Model file for the job. Use its own axes, mm. Coordinates: 2 decimals unless noted, no trailing zeros. Loops run counter-clockwise (first coordinate to the right, second up) from the corner with the lowest first, then second, coordinate; pieces in that order, holes last.
Autodesk Inventor part; units mm, degrees
ref_plane "YZ Plane" through (0, 0, 0) normal (1, 0, 0) x (0, 1, 0)
ref_plane "XZ Plane" through (0, 0, 0) normal (0, 1, 0) x (-1, 0, 0)
ref_plane "XY Plane" through (0, 0, 0) normal (0, 0, 1) x (1, 0, 0)
sketch "Parede_lateral_1" plane through (0, 0, 0) normal (0, 1, 0) x (-1, 0, 0)
  line L0 (0, 0) -> (-95, 0)
  line L1 (-95, 0) -> (-95, -52)
  line L2 (-95, -52) -> (0, -52)
  line L3 (0, -52) -> (0, 0)
  dimension "d0" = 95
  dimension "d1" = 52
extrude "Extrusão1" add sketch "Parede_lateral_1" along normal blind 3
sketch "Esboço4" plane through (0, 3, 0) normal (0, 1, 0) x (1, 0, 0)
  line L0 (0, 52) -> (0, 0)
  line L1 (0, 42) -> (3, 42)
  line L2 (3, 42) -> (3, 32)
  line L3 (3, 32) -> (0, 32)
  line L4 (0, 32) -> (0, 42)
  line L5 (0, 20) -> (3, 20)
  line L6 (3, 20) -> (3, 10)
  line L7 (3, 10) -> (0, 10)
  line L8 (0, 10) -> (0, 20)
  line L9 (95, 0) -> (95, 52)
  line L10 (0, 0) -> (95, 0)
  line L11 (95, 42) -> (92, 42)
  line L12 (92, 42) -> (92, 32)
  line L13 (92, 32) -> (95, 32)
  line L14 (95, 32) -> (95, 42)
  line L15 (95, 20) -> (92, 20)
  line L16 (92, 20) -> (92, 10)
  line L17 (92, 10) -> (95, 10)
  line L18 (95, 10) -> (95, 20)
  line L19 (10, 0) -> (20, 0)
  line L20 (20, 0) -> (20, -3)
  line L21 (20, -3) -> (10, -3)
  line L22 (10, -3) -> (10, 0)
  line L23 (42.5, 0) -> (52.5, 0)
  line L24 (52.5, 0) -> (52.5, -3)
  line L25 (52.5, -3) -> (42.5, -3)
  line L26 (42.5, -3) -> (42.5, 0)
  line L27 (75, 0) -> (85, 0)
  line L28 (85, 0) -> (85, -3)
  line L29 (85, -3) -> (75, -3)
  line L30 (75, -3) -> (75, 0)
  point P0 (1.5, 42)
  point P1 (1.5, 10)
  dimension "d37" = 3
  dimension "d38" = 10
  dimension "d39" = 3
  dimension "d40" = 10
  dimension "d46" = 10
  dimension "d47" = 3
  dimension "d49" = 3
extrude "Extrusão4" add sketch "Esboço4" against normal blind 3 contours L10 L28 L29 L30 | L10 L24 L25 L26 | L10 L20 L21 L22
sketch "Esboço5" plane through (0, 3, 0) normal (0, 1, 0) x (1, 0, 0)
  line L0 (0, 52) -> (0, 0)
  line L1 (0, 10) -> (3, 10)
  line L2 (3, 10) -> (3, 20)
  line L3 (3, 20) -> (0, 20)
  line L4 (0, 20) -> (0, 10)
  line L5 (0, 32) -> (3, 32)
  line L6 (3, 32) -> (3, 42)
  line L7 (3, 42) -> (0, 42)
  line L8 (0, 42) -> (0, 32)
  line L9 (95, 52) -> (0, 52)
  line L10 (0, 0) -> (10, 0)
  line L11 (95, 0) -> (95, 52)
  line L12 (95, 42) -> (92, 42)
  line L13 (92, 42) -> (92, 32)
  line L14 (92, 32) -> (95, 32)
  line L15 (95, 32) -> (95, 42)
  line L16 (95, 20) -> (92, 20)
  line L17 (92, 20) -> (92, 10)
  line L18 (92, 10) -> (95, 10)
  line L19 (95, 10) -> (95, 20)
  point P0 (10, 52)
  point P1 (1.5, 42)
  point P2 (1.5, 10)
  dimension "d52" = 3
  dimension "d53" = 10
  dimension "d54" = 3
  dimension "d55" = 10
  dimension "d56" = 10
  dimension "d57" = 10
  dimension "d58" = 3
extrude "Extrusão5" cut sketch "Esboço5" against normal blind 3
sketch "Esboço17" plane through (0, 3, 0) normal (0, 1, 0) x (1, 0, 0)
  line L0 (53, 35.75) -> (90.5, 35.75)
  line L1 (90.5, 35.75) -> (90.5, 16.25)
  line L2 (90.5, 16.25) -> (53, 16.25)
  line L3 (53, 16.25) -> (53, 35.75)
  line L4 (95, 53) -> (0, 53)
  line L5 (92, 32) -> (92, 42)
  circle A0 centre (90.5, 35.75) radius 0.8
  circle A1 centre (90.5, 16.25) radius 0.8
  circle A2 centre (53, 16.25) radius 0.8
  circle A3 centre (53, 35.75) radius 0.8
  line L6 (85, 0) -> (95, 0)
  line L7 (95, 32) -> (92, 32)
  line L8 (92, 20) -> (95, 20)
  line L9 (52.5, 0) -> (75, 0)
  line L10 (95, 52) -> (0, 52)
  point P0 (0, 0)
  point P1 (90.5, 26)
  point P2 (93.5, 32)
  point P3 (93.5, 20)
  dimension "d130" = 37.5
  dimension "d131" = 19.5
  dimension "d133" = 1.5
  dimension "d134" = 1.6
  dimension "d135" = 1.6
  dimension "d136" = 1.6
  dimension "d137" = 1.6
  dimension "d143" = 3.75
  dimension "d144" = 3.75
  dimension "d146" = 16.25
extrude "Extrusão14" cut sketch "Esboço17" against normal blind 3 contours L3 A3 L0 | L0 A3 L3 | A0 L1 L0 | L0 L1 A0 | A2 L2 L3 | L3 L2 A2 | A1 L2 L1 | L1 L2 A1
sketch "Esboço18" plane through (0, 0, 0) normal (0, -1, 0) x (1, 0, 0)
  line L0 (0, -42) -> (3, -42)
  line L1 (92, -42) -> (92, -32)
  line L2 (92, -42) -> (92, -52)
  line L3 (3, -42) -> (3, -52)
  line L4 (95, -52) -> (0, -52)
  line L5 (3, -52) -> (92, -52)
  line L6 (92, -52) -> (92, -55)
  line L7 (92, -55) -> (3, -55)
  line L8 (3, -55) -> (3, -52)
  point P0 (0, 0)
  dimension "d150" = 3
extrude "Extrusão15" add sketch "Esboço18" against normal blind 3
equation "\"d146\" = -0.5 * d131 + 0.5 * d1"
properties part number "Parede_lateral_3"
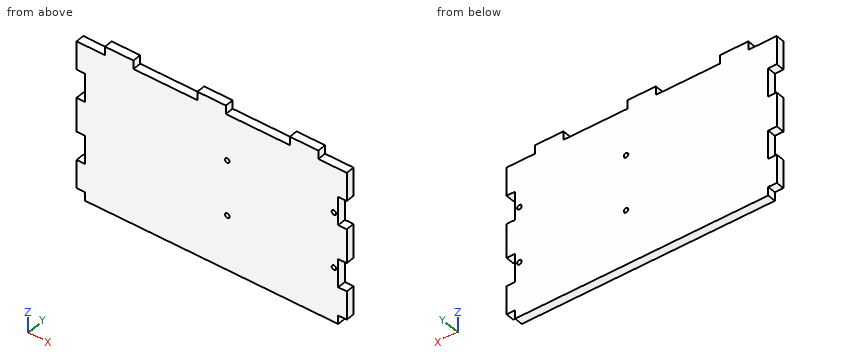
Q1. Slice it at B-B (y = 2.5). Count the separate pieces of the cut face and the enclosed holes in it, and give its area (3 significant figures).
Answers:
separate pieces: 1
enclosed holes: 4
area: 5,170 mm2
Q2. Slice it at A-A (z = -38.5). List the corners of the cut face in (x, y), and give its area (3 significant figures).
Answers:
outline: (3, 0) - (92, 0) - (92, 3) - (3, 3) - close
area: 267 mm2
Q3. Slice it at C-C (x = 28). List the corners of the cut face in (y, z), and give its area (3 significant figures).
Answers:
outline: (0, -55) - (3, -55) - (3, 0) - (0, 0) - close
area: 165 mm2
Q4. Flat gauge pins, fed straight in: P1, Ø1.5, axis at y = 2, z = 1.5, coming from the +X side; P2, Ø2, axis at x = 90.5, z = -35.75, coming from the +Y side; P3, Ø1.5, axis at y = 1, z = -38, coming from the +X side; P4, Ø1.5, axis at x = 59, y = 1, coming from the +Z side. Where does each tip first touch, or does it go through?
Answers:
P1: stops at x = 85
P2: stops at y = 3
P3: stops at x = 92
P4: stops at z = 0
Q5. Drill centre lines: line 1 (Z direction, x = 90.5, y = 1.3); line 2 (X direction, y = 0.7, z = -35.75); line 3 (X direction, y = 0.3, z = -13). Where is each one in solid material? Low to high.
Answers:
line 1: z = -55 to -36.55, -34.95 to -17.05, -15.45 to 0
line 2: x = 3 to 52.2, 53.8 to 89.7, 91.3 to 92
line 3: x = 3 to 92
